Geometry check sheet. Reference: the model listing, model coordinates, mm. Face numbers are marked on the shaded views. A direction names the side the tool comes from. Round coordinates to 2 decimals unless told otherwise and drop trailing zeros. Write each loop counter-clockwise with the first axis right and the second up, starting at its lowest first coordinate (ties: lowest second). Pieces come first, ordered by that corner, then holes. Notation, with made-up numbers: (-5, 10.25) -> (1, 10.25) arc R12 ccw to (1, 23.25) -> close; hole circle Ø8 at (56, 42.5). An arc over 180 degrees is marked (long way). Return JSON: item names as keys, results as strings. Group by question number.
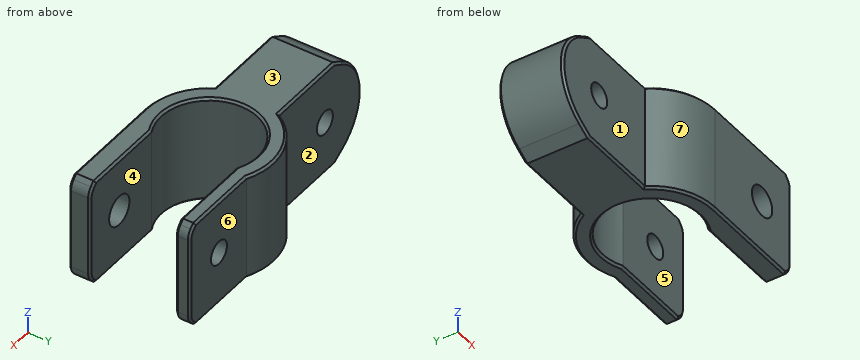
from build123d import *

# Parameters (mm, degrees)
PAD048_DEPTH         = 10
SKETCH195_R          = 2.2
POCKET126_DEPTH      = 12.001
POCKET126_DEPTH_BACK = 12.001
SKETCH238_R          = 2.8
POCKET188_DEPTH      = 4
CHAMFER001_SIZE      = 0.4


with BuildPart() as part:
    # Sketch194 → Pad048 (new body, symmetric)
    with BuildSketch(Plane.XY):
        with BuildLine():
            ThreePointArc((4.123106, 8), (-9, 0), (4.123106, -8))
            Line((4.123106, -8), (21, -8))
            Line((21, -8), (21, -12))
            Line((-3.3e-05, -12), (21, -12))
            ThreePointArc((-10.392305, -6), (-6.000014, -10.392296), (-3.3e-05, -12))
            Line((-33, -6), (-10.392305, -6))
            Line((-33, 6), (-33, -6))
            Line((-10.392305, 6), (-33, 6))
            ThreePointArc((5.497474, 10.666667), (-3.381462, 11.513719), (-10.392305, 6))
            Line((21, 10.666667), (5.497474, 10.666667))
            Line((21, 8), (21, 10.666667))
            Line((4.123106, 8), (21, 8))
        make_face()
    extrude(amount=PAD048_DEPTH, both=True)

    # Sketch195 → Pocket126 (cut, two sides)
    with BuildSketch(Plane.XZ) as pocket126_sk:
        with Locations((13, 0)):
            Circle(SKETCH195_R)
        with Locations((-23, 0)):
            Circle(SKETCH195_R)
        with BuildLine():
            ThreePointArc((-28, 8.660254), (-33, 0), (-28, -8.660254))
            Line((-28, -8.660254), (-25.679492, -10))
            Line((-25.679492, -10), (-25.679492, -11))
            Line((-25.679492, -11), (-34, -11))
            Line((-34, -11), (-34, 11))
            Line((-34, 11), (-25.679492, 11))
            Line((-25.679492, 11), (-25.679492, 10))
            Line((-28, 8.660254), (-25.679492, 10))
        make_face()
        with BuildLine():
            ThreePointArc((21, 7.5), (20.809699, 8.456709), (20.267767, 9.267767))
            Line((19.535534, 10), (20.267767, 9.267767))
            Line((19.535534, 10), (19.535534, 11))
            Line((19.535534, 11), (22, 11))
            Line((22, 11), (22, -11))
            Line((22, -11), (19.535534, -11))
            Line((19.535534, -11), (19.535534, -10))
            Line((19.535534, -10), (20.267767, -9.267767))
            ThreePointArc((20.267767, -9.267767), (20.809699, -8.456709), (21, -7.5))
            Line((21, -7.5), (21, 7.5))
        make_face()
    extrude(amount=-POCKET126_DEPTH, mode=Mode.SUBTRACT)
    extrude(pocket126_sk.sketch, amount=POCKET126_DEPTH_BACK, mode=Mode.SUBTRACT)

    # Sketch238 (on DatumPlane) → Pocket188 (cut)
    with BuildSketch(Plane(origin=(13, -12, 0), x_dir=(0, 0, 1), z_dir=(0, -1, 0))):
        Circle(SKETCH238_R)
    extrude(amount=-POCKET188_DEPTH, mode=Mode.SUBTRACT)

    # Chamfer001
    chamfer001_edges = [part.edges().sort_by_distance(p)[0] for p in [
        (-18.035898, 6, 10),
        (-18.035898, -6, 10),
        (-6.000014, -10.392296, 10),
        (9.76775, -12, 10),
        (-9, 0, 10),
        (11.82932, -8, 10),
        (11.82932, 8, 10),
        (12.516504, 10.666667, 10),
        (-3.381462, 11.513719, 10),
        (12.516504, 10.666667, -10),
        (11.82932, 8, -10),
        (-3.381462, 11.513719, -10),
        (-9, 0, -10),
        (11.82932, -8, -10),
        (9.76775, -12, -10),
        (-6.000014, -10.392296, -10),
        (-18.035898, -6, -10),
        (-18.035898, 6, -10),
        (-26.839746, 6, 9.330127),
        (-31.660254, 6, 5),
        (-31.660254, 6, -5),
        (-26.839746, 6, -9.330127),
        (-26.839746, -6, 9.330127),
        (-31.660254, -6, 5),
        (-31.660254, -6, -5),
        (-26.839746, -6, -9.330127),
        (19.90165, -12, 9.633883),
        (20.809699, -12, 8.456709),
        (21, -12, 0),
        (20.809699, -12, -8.456709),
        (19.90165, -12, -9.633883),
        (19.90165, -8, 9.633883),
        (20.809699, -8, 8.456709),
        (21, -8, 0),
        (20.809699, -8, -8.456709),
        (19.90165, -8, -9.633883),
        (19.90165, 8, -9.633883),
        (19.90165, 10.666667, -9.633883),
        (20.809699, 10.666667, -8.456709),
        (20.809699, 8, -8.456709),
        (21, 10.666667, 0),
        (21, 8, 0),
        (20.809699, 10.666667, 8.456709),
        (19.90165, 10.666667, 9.633883),
        (19.90165, 8, 9.633883),
        (20.809699, 8, 8.456709),
    ]]
    chamfer(chamfer001_edges, length=CHAMFER001_SIZE)


with BuildPart() as part_1:
    # Body022042 placement: moved
    add(part.part.moved(Location((113, -113, 428.30889))))


solid = part_1.part
1) Sectioned sample at B-B on x = 102. Enter the section's corners in (y, z), and give its area (3 significant figures).
2) Mould release check, pull along Y, two halves, no side actions. Record for the marked faces 4, 5, 6 and 7: +Y half, -Y half, draft (parallel to the pull), parting line (faces both ways), or undercut.
3) Sectioned sample at A-A on x = 90. Enter the section's corners in (y, z).
4) Material ranges on probe 1 along Y at (x, z) = (129.5, 421.25); probe 2 along Z at (x, y) = (90, -116.25); probe 3 along Z at (x, y) = (126, -122.5), recorded low to high. Write a range as [from, to].
5) Go/stop test with flat-tipped pins: P1, Ø2, axis at x = 92.5, z = 431, coming from the +Y side; P2, Ø8, axis at x = 108.5, y = -113, coming from the -Z side; P3, Ø9.5, axis at x = 86.5, z = 424, coming from the -Y side; P4, Ø4.5, axis at x = 126, z = 428.31, coming from the -Y side. Record where each tip stops, or that it passes through.
6) Tool access check on the marked faces 1, 2 and 3. Record the directions out of +Z, -Z, +X, -X, +Y, -Y that give a thin tool (end or side, any length) a straight path to the whole face; none if there is none.
7) Sectioned sample at D-D on x = 121.5. Enter the section's corners in (y, z), and give its area (3 significant figures).
8) Sectioned sample at C-C on y = -113. Enter the section's corners in (x, z).
Evaluation:
{
 "1": {"outline": "(-119, 418.71) -> (-118.6, 418.31) -> (-107.4, 418.31) -> (-107, 418.71) -> (-107, 437.91) -> (-107.4, 438.31) -> (-118.6, 438.31) -> (-119, 437.91) -> close", "area": "240 mm2"},
 "2": {"face 4": "undercut", "face 5": "undercut", "face 6": "+Y half", "face 7": "-Y half"},
 "3": {"outline": "(-119, 418.71) -> (-118.6, 418.31) -> (-107.4, 418.31) -> (-107, 418.71) -> (-107, 426.11) -> (-119, 426.11) -> close; (-119, 430.51) -> (-107, 430.51) -> (-107, 437.91) -> (-107.4, 438.31) -> (-118.6, 438.31) -> (-119, 437.91) -> close"},
 "4": {"probe 1": "y = [-125, -121], [-105, -102.33]", "probe 2": "z = [418.31, 426.11], [430.51, 438.31]", "probe 3": "z = [418.31, 425.51], [431.11, 438.31]"},
 "5": {"P1": "stops at y = -107", "P2": "passes through", "P3": "stops at y = -119", "P4": "stops at y = -105"},
 "6": {"face 1": "+Z, -Z, -X, -Y", "face 2": "+Z, -Z, -X, +Y", "face 3": "+Z, +X, -X, +Y, -Y"},
 "7": {"outline": "(-125, 418.71) -> (-124.6, 418.31) -> (-121.4, 418.31) -> (-121, 418.71) -> (-121, 437.91) -> (-121.4, 438.31) -> (-124.6, 438.31) -> (-125, 437.91) -> close; (-105, 418.71) -> (-104.6, 418.31) -> (-102.73, 418.31) -> (-102.33, 418.71) -> (-102.33, 437.91) -> (-102.73, 438.31) -> (-104.6, 438.31) -> (-105, 437.91) -> close", "area": "133 mm2"},
 "8": {"outline": "(85, 419.65) -> (87.32, 418.31) -> (103.6, 418.31) -> (104, 418.71) -> (104, 437.91) -> (103.6, 438.31) -> (87.32, 438.31) -> (85, 436.97) arc R10 ccw to start; hole circle Ø4.4 at (90, 428.31)"}
}
